from build123d import *

# Parameters (mm, degrees)
ESQUISSE2_W             = 13
ESQUISSE2_H             = 171
BOSS_EXTRU_1_DEPTH      = 13
BOSS_EXTRU_2_DEPTH      = 13
ESQUISSE4_W             = 11
ESQUISSE4_H             = 12
ENL_V_MAT_EXTRU_2_DEPTH = 37


with BuildPart() as part:
    # Esquisse2 → Boss.-Extru.1 (new body)
    with BuildSketch(Plane.XY):
        with Locations((-64.835362299, 95.5)):
            Rectangle(ESQUISSE2_W, ESQUISSE2_H)
    extrude(amount=BOSS_EXTRU_1_DEPTH)

    # Esquisse2<3> → Boss.-Extru.2 (add)
    with BuildSketch(Plane.XY):
        Polygon((-58.335362299, 10), (-71.335362299, 10), (-71.335362299, 0), (13.664637701, 0), (13.664637701, 10), align=None)
    extrude(amount=BOSS_EXTRU_2_DEPTH)

    # Esquisse4 → Enlèv. mat.-Extru.2 (cut)
    with BuildSketch(Plane(origin=(-58.335362299, 0, 0), x_dir=(0, 0, -1), z_dir=(1, 0, 0))):
        with Locations((-6.5, 61)):
            Rectangle(ESQUISSE4_W, ESQUISSE4_H)
    extrude(amount=-ENL_V_MAT_EXTRU_2_DEPTH, mode=Mode.SUBTRACT)


solid = part.part
Read the model definition and answer for the solid it produces. Units are mm, in the model's axes. A direction names the side the tool comes from. Give positions to 0.01 mm unless a question says otherwise; leave off trailing zeros. Loops run counter-clockwise (first coordinate to the right, second up) from the corner with the lowest first, then second, coordinate; pieces in that order, holes last. Notation, with made-up numbers: (27.5, 16.25) - (62.5, 16.25) arc R17 cw to (62.5, 24.25) - close; hole circle Ø3 at (13.5, 5.5). An arc over 180 degrees is marked (long way). Answer as CSV lines item,"result". Start each with the question number.
1) Each of these flat-tipped pins is pushed along its axis until it touches: pin 1 Ø5 at (x, z) = (-8.5, 7) entering from +Y; pin 2 Ø6.5 at (y, z) = (58.5, 3.5) entering from +X. Where does it stop, or does it pass through?
2) Straight lines are drawn through the part: L1, parallel to Y at x = -59, z = 4.75; L2, parallel to X at y = 45, z = 3.75; L3, parallel to Y at x = -34, z = 11.25. For each, find the intervals that lie inside material, in ascending order. Write a range as from..to.
3) Determine the mould class of faces 1 (the face through (-61, 78, 13)), 2 (the face through (-65, 61, 12)), 3 (the face through (-65, 181, 6)) for opening direction Y: released by +Y, released by -Y, zero draft, split by the parting line, or undercut.
4) Find section A-A (z = 9). Write down the section's boundary in (x, y), then the cut area to 3 significant figures.
5) Which of the six approach directions +Z, -Z, +X, -X, +Y, -Y give full straight-line access (tool end or side, diameter ignored) to faces 4 (the face through (-29, 0, 6)), 5 (the face through (-58.335, 94, 6)), 6 (the face through (-65, 67, 7))?
6) Find section C-C (y = 73). Write down the section's boundary in (x, z).
7) Find section B-B (x = -21). Write down the section's boundary in (y, z).
Findings below:
1,pin 1,"y = 10"
1,pin 2,"x = -58.34"
2,L1,"0..55, 67..181"
2,L2,"-71.34..-58.34"
2,L3,"0..10"
3,face 1,"zero draft"
3,face 2,"undercut"
3,face 3,"released by +Y"
4,outline,"(-71.34, 0) - (13.66, 0) - (13.66, 10) - (-58.34, 10) - (-58.34, 55) - (-71.34, 55) - close; (-71.34, 67) - (-58.34, 67) - (-58.34, 181) - (-71.34, 181) - close"
4,area,"2,920 mm^2"
5,face 4,"+Z, -Z, +X, -X, -Y"
5,face 5,"+Z, -Z, +X, +Y"
5,face 6,"+X, -X"
6,outline,"(-71.34, 0) - (-58.34, 0) - (-58.34, 13) - (-71.34, 13) - close"
7,outline,"(0, 0) - (10, 0) - (10, 13) - (0, 13) - close"
